Build history of the part. All positions in model axes, mm. Face numbers are marked on the shaded views. A direction names the side the tool comes from. Coordinates: 2 decimals unless noted, no trailing zeros. Write each loop counter-clockwise with the first axis right and the second up, starting at its lowest first coordinate (ties: lowest second). Pieces come first, ordered by that corner, then holes. Notation, with made-up numbers: M -24,28.25 L 18,28.25 A26 ccw 18,54.25 Z; hole C -38,46 d7. An arc over 180 degrees is marked long. Use CSV: the item, a comma, the result in double quotes. Start each with the question number.
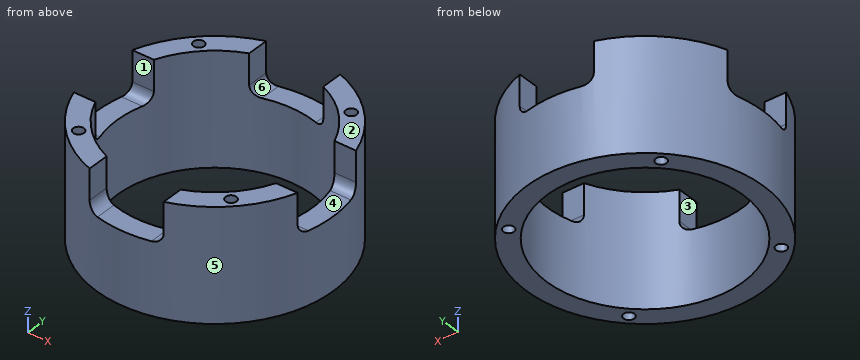
```python
from build123d import *

# Parameters (mm, degrees)
SKETCH_1_R          = 35
SKETCH_1_R_2        = 29
SKETCH_1_R_3        = 1.6
EXTRUDE_1_DEPTH     = 33.2
SKETCH_3_W          = 22
SKETCH_3_H          = 23.089675748
SKETCH_3_W_2        = 23.089675748
SKETCH_3_H_2        = 22
CUT_EXTRUDE_1_DEPTH = 12
FILLET_1_R          = 3


with BuildPart() as part:
    # 草图1 → 凸台-拉伸1 (new body)
    with BuildSketch(Plane.XY):
        with Locations(Location((0, 0, 0), (0, 0, 180))):
            Circle(SKETCH_1_R)
        with Locations(Location((0, 0, 0), (0, 0, 180))):
            Circle(SKETCH_1_R_2, mode=Mode.SUBTRACT)
        with Locations(Location((-22.627416998, 22.627416998, 0), (0, 0, 180))):
            Circle(SKETCH_1_R_3, mode=Mode.SUBTRACT)
        with Locations(Location((22.627416998, 22.627416998, 0), (0, 0, 180))):
            Circle(SKETCH_1_R_3, mode=Mode.SUBTRACT)
        with Locations(Location((22.627416998, -22.627416998, 0), (0, 0, 180))):
            Circle(SKETCH_1_R_3, mode=Mode.SUBTRACT)
        with Locations(Location((-22.627416998, -22.627416998, 0), (0, 0, 180))):
            Circle(SKETCH_1_R_3, mode=Mode.SUBTRACT)
    extrude(amount=EXTRUDE_1_DEPTH)

    # 草图3 → 切除-拉伸1 (cut)
    with BuildSketch(Plane.XY.offset(33.2)):
        with Locations((0, 32.883523325)):
            Rectangle(SKETCH_3_W, SKETCH_3_H)
        with Locations((32.883523325, 0)):
            Rectangle(SKETCH_3_W_2, SKETCH_3_H_2)
        with Locations((0, -32.883523325)):
            Rectangle(SKETCH_3_W, SKETCH_3_H)
        with Locations((-32.883523325, 0)):
            Rectangle(SKETCH_3_W_2, SKETCH_3_H_2)
    extrude(amount=-CUT_EXTRUDE_1_DEPTH, mode=Mode.SUBTRACT)

    # 圆角1
    fillet_1_edges = [part.edges().sort_by_distance(p)[0] for p in [
        (-11, 30.029655591, 21.2),
        (11, 30.029655591, 21.2),
        (30.029655591, 11, 21.2),
        (30.029655591, -11, 21.2),
        (11, -30.029655591, 21.2),
        (-11, -30.029655591, 21.2),
        (-30.029655591, -11, 21.2),
        (-30.029655591, 11, 21.2),
    ]]
    fillet(fillet_1_edges, radius=FILLET_1_R)


solid = part.part
```
1. Flat gauge pins, fed straight in: pin 1 (1.5 mm diameter, centred on y = 14.5, z = 22.5, fed in from +X); pin 2 (1 mm diameter, centred on y = 0.5, z = 13.5, fed in from -X); pin 3 (6 mm diameter, centred on y = 23.5, z = 28.5, fed in from +X); pin 4 (6 mm diameter, centred on y = 19.5, z = 9, fed in from +X). Where does each tip first touch, or does it go through?
2. Drill centre lines: line 1 along X through (y, z) = (1, 15.5); line 2 along Y through (x, z) = (0, 9); line 3 along X through (y, z) = (-20.5, 3). Where is each one in solid material? Low to high. Write a range as from..to.
3. Slice it at D-D (x = -23). List the corners of the cut face in (y, z).
4. Slice it at A-A (x = 0). List the corners of the cut face in (y, z).
5. 3-axis set-ups, long thin cutter, end or side, ignore diameter. For the marked faces 1, 2 and 3: which of +Z, -Z, +X, -X, +Y, -Y reach the whole face in a straight line?
6. Pull direction X, two halves, no side cores. Call the marked faces 4, 5 and 6: pulls with the +X half, pulls with the -X half, needs draft (parallel to the pull), parting line crosses it, or undercut.
7. Slice it at C-C (z = 28). List the corners of the cut face in (x, y).
Established:
1,pin 1,"stops at x = 32.19"
1,pin 2,"stops at x = -35"
1,pin 3,"stops at x = 28.37"
1,pin 4,"stops at x = 30.87"
2,line 1,"x = -34.99..-28.98, 28.98..34.99"
2,line 2,"y = -35..-29, 29..35"
2,line 3,"x = -28.37..-20.51, 20.51..28.37"
3,outline,"M -26.38,0 L -24.18,0 L -24.18,33.2 L -26.38,33.2 Z; M -21.07,0 L -17.66,0 L -17.66,33.2 L -21.07,33.2 Z; M 17.66,0 L 21.07,0 L 21.07,33.2 L 17.66,33.2 Z; M 24.18,0 L 26.38,0 L 26.38,33.2 L 24.18,33.2 Z"
4,outline,"M -35,0 L -29,0 L -29,21.2 L -35,21.2 Z; M 29,0 L 35,0 L 35,21.2 L 29,21.2 Z"
5,face 1,"+Z, +X, -X"
5,face 2,"+Z, +X, -X, +Y, -Y"
5,face 3,"+Z, +Y, -Y"
6,face 4,"needs draft"
6,face 5,"parting line crosses it"
6,face 6,"undercut"
7,outline,"M -33.23,-11 A35 ccw -11,-33.23 L -11,-26.83 A29 cw -26.83,-11 Z; M -33.23,11 L -26.83,11 A29 cw -11,26.83 L -11,33.23 A35 ccw Z; M 11,-33.23 A35 ccw 33.23,-11 L 26.83,-11 A29 cw 11,-26.83 Z; M 11,26.83 A29 cw 26.83,11 L 33.23,11 A35 ccw 11,33.23 Z; hole C -22.63,-22.63 d3.2; hole C -22.63,22.63 d3.2; hole C 22.63,-22.63 d3.2; hole C 22.63,22.63 d3.2"
